```python
from build123d import *

# Parameters (mm, degrees)
F0_W      = 850.9
F0_H      = 673.1
F1_DEPTH  = 304.8
F2_T      = -3.175
F3_W      = 584.2
F3_H      = 101.6
F4_DEPTH  = 558.8
F5_W      = 431.8
F5_H      = 69.85
F6_DEPTH  = 25.4
F7_T      = -2.54
F8_R      = 6.35
F9_DEPTH  = 2.54
F10_W     = 927.1
F10_H     = 749.3
F10_W_2   = 850.9
F10_H_2   = 673.1
F11_DEPTH = 3.175
F12_R     = 6.35
F13_R     = 6.35
F15_DEPTH = 584.2


# Not quite as in the source:
# - a shell that OpenCascade refuses in one call is made with other operations: the cavity is built on its own and cut out


with BuildPart() as f1:
    # F0 (on Top) → F1 (new body)
    with BuildSketch(Plane.XY):
        Rectangle(F0_W, F0_H)
    extrude(amount=F1_DEPTH)

    # F2
    f2_openings = [f1.faces().sort_by_distance(p)[0] for p in [
        (0, 0, 304.8),
    ]]
    offset(amount=F2_T, openings=f2_openings)

    # F3 (on face) → F4 (join)
    with BuildSketch(Plane.XZ.offset(-333.375)):
        with Locations((79.3750111103, 53.975)):
            Rectangle(F3_W, F3_H)
    extrude(amount=F4_DEPTH)

    # F5 (on face) → F6 (cut)
    with BuildSketch(Plane.XZ.offset(225.425)):
        with Locations((79.3750111103, 38.1)):
            Rectangle(F5_W, F5_H)
    extrude(amount=-F6_DEPTH, mode=Mode.SUBTRACT)

    # F7: a shell. OpenCascade refuses it in one call, so the cavity is built on its own and cut out:
    # the body offset inwards by the wall thickness, plus a prism from it out through each open face.
    f7_core = offset(f1.part, amount=F7_T, kind=Kind.INTERSECTION, mode=Mode.PRIVATE)
    f7_exits = [f7_core.faces().sort_by_distance(p)[0] for p in [
        (303.691397, -222.885, 39.0525),
    ]]
    add(f7_core, mode=Mode.SUBTRACT)
    extrude(f7_exits, amount=-F7_T, mode=Mode.SUBTRACT)

    # F8 (on face) → F9 (cut, through all)
    with BuildSketch(Plane.XY.offset(104.775)):
        with Locations((219.0750111103, 269.875)):
            Circle(F8_R)
        with Locations((-60.3249888897, 269.875)):
            Circle(F8_R)
        with Locations((-60.3249888897, -161.925)):
            Circle(F8_R)
        with Locations((219.0750111103, -161.925)):
            Circle(F8_R)
    extrude(amount=-F9_DEPTH, mode=Mode.SUBTRACT)

    # F10 (on face) → F11 (join)
    with BuildSketch(Plane.XY.offset(304.8)):
        Rectangle(F10_W, F10_H)
        Rectangle(F10_W_2, F10_H_2, mode=Mode.SUBTRACT)
    extrude(amount=-F11_DEPTH)

    # F12
    f12_edges = [f1.edges().sort_by_distance(p)[0] for p in [
        (0, -336.55, 0),
    ]]
    fillet(f12_edges, radius=F12_R)

    # F13
    f13_edges = [f1.edges().sort_by_distance(p)[0] for p in [
        (0, 336.55, 0),
    ]]
    fillet(f13_edges, radius=F13_R)

    # F14 (on face) → F15 (cut, through all)
    with BuildSketch(Plane(origin=(-212.7249888897, 0, 0), x_dir=(0, -1, 0), z_dir=(-1, 0, 0))):
        with BuildLine():
            ThreePointArc((-254.2258527756, 3.175), (-277.4081012725, 59.1418987275), (-333.375, 82.3241472244))
            Line((-333.375, 82.3241472244), (-333.375, 3.175))
            Line((-333.375, 3.175), (-254.2258527756, 3.175))
        make_face()
    extrude(amount=-F15_DEPTH, mode=Mode.SUBTRACT)


solid = f1.part
```
Verification items for the finished model (mm, model axes). A direction names the side the tool comes from. Coordinates: 2 decimals unless noted, no trailing zeros. Loops run counter-clockwise (first coordinate to the right, second up) from the corner with the lowest first, then second, coordinate; pieces in that order, holes last. Notation, with made-up numbers: (31, 36) -> (80, 36) arc R15 cw to (80, 52) -> close; hole circle Ø7 at (-1, 53). An arc over 180 degrees is marked (long way). Put each result on its own line as item: value.
1. Gauge pin test, flat ends, axial feed: P1, Ø10, axis at y = 288.5, z = 131.5, coming from the -X side; P2, Ø5, axis at x = 216, z = 107.5, coming from the -Y side; P3, Ø3, axis at x = 187.5, y = -289.5, coming from the +Z side (3 decimals). Record the tip position at first contact, or that the pin passes through.
Result set:
P1: stops at x = -425.45
P2: stops at y = -336.55
P3: stops at z = 3.175
2. Section check B-B, the plane z = 35. Record the boundary of the cut face in (x, y) (3 decimals), then the cut area to 3 significant figures.
Result set:
outline: (-425.45, -336.55) -> (425.45, -336.55) -> (425.45, 336.55) -> (-425.45, 336.55) -> close; (-212.725, -225.425) -> (-210.185, -225.425) -> (-210.185, 260.906) -> (-212.725, 260.906) -> close; (-139.065, -225.425) -> (-136.525, -225.425) -> (-136.525, -200.025) -> (295.275, -200.025) -> (295.275, -225.425) -> (297.815, -225.425) -> (297.815, -197.485) -> (-139.065, -197.485) -> close; (368.935, -225.425) -> (371.475, -225.425) -> (371.475, 260.906) -> (368.935, 260.906) -> close; hole (-422.275, -333.375) -> (422.275, -333.375) -> (422.275, 333.375) -> (368.935, 333.375) -> (368.935, 334.01) -> (-210.185, 334.01) -> (-210.185, 333.375) -> (-422.275, 333.375) -> close
area: 13,000 mm^2
3. Section check D-D, the plane z = 148. Record the boundary of the cut face in (x, y) (3 decimals).
Result set:
outline: (-425.45, -336.55) -> (425.45, -336.55) -> (425.45, 336.55) -> (-425.45, 336.55) -> close; hole (-422.275, -333.375) -> (422.275, -333.375) -> (422.275, 333.375) -> (-422.275, 333.375) -> close
4. Section check C-C, the plane x = 329.5. Record the boundary of the cut face in (y, z) (3 decimals).
Result set:
outline: (-374.65, 301.625) -> (-336.55, 301.625) -> (-336.55, 6.35) arc R6.35 ccw to (-330.2, 0) -> (330.2, 0) arc R6.35 ccw to (336.55, 6.35) -> (336.55, 301.625) -> (374.65, 301.625) -> (374.65, 304.8) -> (333.375, 304.8) -> (333.375, 104.775) -> (-225.425, 104.775) -> (-225.425, 102.235) -> (334.01, 102.235) -> (334.01, 2.54) -> (-225.425, 2.54) -> (-225.425, 3.175) -> (-333.375, 3.175) -> (-333.375, 304.8) -> (-374.65, 304.8) -> close
5. Thickness scan on line 1 (Y direction, x = 267, z = 25) (3 decimals); line 2 (X direction, y = 198, z = 34) (3 decimals); line 3 (Y direction, x = 414.5, z = 233) (3 decimals). Record the ranges inside material, lowest first.
Result set:
line 1: y = -336.55 to -333.375, -200.025 to -197.485, 334.01 to 336.55
line 2: x = -425.45 to -422.275, -212.725 to -210.185, 368.935 to 371.475, 422.275 to 425.45
line 3: y = -336.55 to -333.375, 333.375 to 336.55
6. Tool access check on faces 1 (the face through (-6, 5, 0)), 2 (the face through (370.187, 276.796, 58.523)), 3 (the face through (78, -225.425, 103)). Record the directions out of +Z, -Z, +X, -X, +Y, -Y that give a thin tool (end or side, any length) a straight path to the whole face; none if there is none.
Result set:
face 1: -Z, +X, -X, +Y, -Y
face 2: none
face 3: +Z
7. Section check A-A, the plane y = -96.5. Record the boundary of the cut face in (x, z) (3 decimals), then the cut area to 3 significant figures.
Result set:
outline: (-463.55, 301.625) -> (-425.45, 301.625) -> (-425.45, 0) -> (425.45, 0) -> (425.45, 301.625) -> (463.55, 301.625) -> (463.55, 304.8) -> (422.275, 304.8) -> (422.275, 3.175) -> (371.475, 3.175) -> (371.475, 104.775) -> (-212.725, 104.775) -> (-212.725, 3.175) -> (-422.275, 3.175) -> (-422.275, 304.8) -> (-463.55, 304.8) -> close; hole (-210.185, 2.54) -> (368.935, 2.54) -> (368.935, 102.235) -> (-210.185, 102.235) -> close
area: 6,480 mm^2
8. Mould release check, pull along Y, two halves, no side actions. Record for faces 4 (the face through (-37, -359, 301.625)), 5 (the face through (76, -213, 73.025)), 6 (the face through (-6, 336.55, 152)): pulls with the +Y half, pulls with the -Y half, needs draft (parallel to the pull), parting line crosses it, or undercut.
Result set:
face 4: needs draft
face 5: undercut
face 6: pulls with the +Y half
